The listing builds one solid part. Answer for the finished solid, in the listing's coordinates (mm). A direction names the side the tool comes from. Coordinates: 2 decimals unless noted, no trailing zeros. Order: outer loops, then holes, each group sorted by start corner. A loop starts at its lowest first (then second) coordinate and runs counter-clockwise, first axis right, second up. Notation, with made-up numbers: (61.5, 6) -> (81.5, 6) arc R14 ccw to (81.5, 19) -> close; hole circle Ø11 at (66, 7.25). An arc over 180 degrees is marked (long way). Put each result on its own line as item: value. Start each with the question number.
```python
from build123d import *

# Parameters (mm, degrees)
SKETCH_1_R              = 6.65
EXTRUDE_1_DEPTH         = 1.25
EXTRUDE_2_DEPTH         = 1.25
EXTRUDE_2_DEPTH_BACK    = 7
SKETCH_3_R              = 1.1
CUT_EXTRUDE_1_DEPTH     = 5
CHAMFER_1_SIZE          = 0.7
CUT_EXTRUDE1_DEPTH      = 10
CUT_EXTRUDE1_DEPTH_BACK = 10
SKETCH1_W               = 17.169793681
SKETCH1_H               = 8.928336681


with BuildPart() as part:
    # Эскиз1 → Бобышка-Вытянуть1 (new, symmetric)
    with BuildSketch(Plane(origin=(0, 0, 0), x_dir=(0, 0, -1), z_dir=(1, 0, 0))):
        with BuildLine():
            Line((-31.25, 0), (-10, 0))
            ThreePointArc((-10, 0), (-2.588190451, -9.659258263), (8.660254038, -5))
            Line((8.660254038, -5), (76.721847542, -5))
            ThreePointArc((76.721847542, -5), (75.425886146, -4.389181279), (74.09117429, -3.868451302))
            ThreePointArc((74.09117429, -3.868451302), (74.147561595, -2.912548148), (74.149130868, -1.954984622))
            ThreePointArc((74.149130868, -1.954984622), (75.638846987, -1.51744657), (77.087831178, -0.959648686))
            ThreePointArc((77.087831178, -0.959648686), (77.109856091, -0.006099484), (77.083941958, 0.947351948))
            ThreePointArc((77.083941958, 0.947351948), (75.643750299, 1.505844774), (74.166291118, 1.956600379))
            ThreePointArc((74.166291118, 1.956600379), (74.147505302, 2.913980899), (74.073940169, 3.8687157))
            ThreePointArc((74.073940169, 3.8687157), (75.433826566, 4.383081961), (76.750365892, 5))
            Line((76.750365892, 5), (8.660254038, 5))
            ThreePointArc((8.660254038, 5), (5, 8.660254038), (0, 10))
            Line((0, 10), (-34.75, 10))
            Line((-34.75, 10), (-34.75, 5))
            Line((-34.75, 5), (-35.25, 5))
            Line((-35.25, 5), (-35.25, 4))
            ThreePointArc((-35.25, 4), (-34.078427125, 1.171572875), (-31.25, 0))
        make_face()
        Circle(SKETCH_1_R, mode=Mode.SUBTRACT)
    extrude(amount=EXTRUDE_1_DEPTH, both=True)

    # Эскиз1<5> → Бобышка-Вытянуть2 (add, two sides: drawn at the far end of the back side and taken through both)
    with BuildSketch(Plane(origin=(0, 0, 0), x_dir=(0, 0, -1), z_dir=(1, 0, 0)).offset(-EXTRUDE_2_DEPTH_BACK)):
        with BuildLine():
            Line((73.559260736, 9.685830974), (74.227172899, 10))
            Line((74.227172899, 10), (80.32185029, 10))
            ThreePointArc((80.32185029, 10), (80.927765714, -1.515378033), (79.891173693, -13))
            Line((79.891173693, -13), (75.988629927, -13.007027449))
            ThreePointArc((75.988629927, -13.007027449), (76.159551637, -12.068663477), (76.283109214, -11.12289675))
            ThreePointArc((76.283109214, -11.12289675), (74.948016231, -10.345984286), (73.559260736, -9.669652694))
            ThreePointArc((73.559260736, -9.669652694), (73.690473514, -8.721120367), (73.767167518, -7.766631814))
            ThreePointArc((73.767167518, -7.766631814), (75.28662018, -7.447324325), (76.774901953, -7.004931935))
            ThreePointArc((76.774901953, -7.004931935), (76.871673579, -6.056050262), (76.920646267, -5.103504803))
            ThreePointArc((76.920646267, -5.103504803), (75.528713081, -4.433737489), (74.09117429, -3.868451302))
            ThreePointArc((74.09117429, -3.868451302), (74.147561595, -2.912548148), (74.149130868, -1.954984622))
            ThreePointArc((74.149130868, -1.954984622), (75.638846987, -1.51744657), (77.087831178, -0.959648686))
            ThreePointArc((77.087831178, -0.959648686), (77.109856091, -0.006099484), (77.083941958, 0.947351948))
            ThreePointArc((77.083941958, 0.947351948), (75.643750299, 1.505844774), (74.166291118, 1.956600379))
            ThreePointArc((74.166291118, 1.956600379), (74.147505302, 2.913980899), (74.073940169, 3.8687157))
            ThreePointArc((74.073940169, 3.8687157), (75.524735151, 4.421786748), (76.925488289, 5.091551117))
            ThreePointArc((76.925488289, 5.091551117), (76.872630699, 6.043888899), (76.771989513, 6.992367959))
            ThreePointArc((76.771989513, 6.992367959), (75.292418643, 7.436143003), (73.784148097, 7.769588967))
            ThreePointArc((73.784148097, 7.769588967), (73.691130431, 8.729989779), (73.559260736, 9.685830974))
        make_face()
    extrude(amount=EXTRUDE_2_DEPTH + EXTRUDE_2_DEPTH_BACK)

    # Эскиз3 → Вырез-Вытянуть1 (cut)
    with BuildSketch(Plane(origin=(0, 10, 0), x_dir=(1, 0, 0), z_dir=(0, 1, 0))):
        with Locations((0, -35)):
            Circle(SKETCH_3_R)
    extrude(amount=-CUT_EXTRUDE_1_DEPTH, mode=Mode.SUBTRACT)

    # Фаска1
    chamfer_1_edges = [part.edges().sort_by_distance(p)[0] for p in [
        (-1.25, 0, 6.65),
    ]]
    chamfer(chamfer_1_edges, length=CHAMFER_1_SIZE)

    # Sketch1 → Cut-Extrude1 (cut, two sides: drawn at the far end of the back side and taken through both)
    with BuildSketch(Plane(origin=(0, 0, 0), x_dir=(0, 0, -1), z_dir=(1, 0, 0)).offset(-CUT_EXTRUDE1_DEPTH_BACK)):
        with Locations((77.607372566, 9.464168341)):
            Rectangle(SKETCH1_W, SKETCH1_H)
    extrude(amount=CUT_EXTRUDE1_DEPTH + CUT_EXTRUDE1_DEPTH_BACK, mode=Mode.SUBTRACT)


solid = part.part
```
(1) A tool of negligible diameter and unlimited length cuts with its end or side. For faces 1 (the cylindrical face through (-2.93, -6.07, -76.87)), 2 (the cylindrical face through (-4.165, 4.375, -75.415)), 3 (the flat face through (0, 0, 21)), from which of +Z, -Z, +X, -X, +Y, -Y can it reach the whole face along a straight path? Write none if from no direction.
(2) The part is cut by section B-B on z = -66.5. Determine the outline of the cut face in (x, y), plus the area to 3 significant figures.
(3) Each of these flat-tipped pins is pushed along its axis until it touches: P1, Ø1.2, axis at x = 0.5, z = 21.5, coming from the -Y side; P2, Ø6, axis at y = -1, z = -24, coming from the -X side; P3, Ø1.2, axis at x = 0, z = -52, coming from the -Y side. Where does it stop, or does it pass through?
(4) The part is cut by section A-A on x = -5.5. Determine the outline of the cut face in (y, z).
(5) Find the intervals of material crossed by L1, parallel to X at y = 1.5, z = 25.5; L2, parallel to Y at x = 0.25, z = 13; L3, parallel to Z at x = -2.75, y = 0.25, in increasing order.
(6) For a pull along Y with two mould halves and no side action, classify faces 4 (the cylindrical face through (-2.93, -8.73, -73.69)), 5 (the flat face through (-1, 5, -47)), 6 (the cylindrical face through (0, 7.5, 33.9)) as released by +Y, released by -Y, zero draft, split by the parting line, or undercut.
Worked out:
1. face 1: +X, -X
1. face 2: +Z, -X, +Y
1. face 3: +Z, +X, -X, -Y
2. outline: (-1.25, -5) -> (1.25, -5) -> (1.25, 5) -> (-1.25, 5) -> close
2. area: 25.0 mm2
3. P1: y = 0
3. P2: x = -1.25
3. P3: y = -5
4. outline: (-13.01, -75.99) -> (-13, -79.89) arc R80.94 ccw to (5, -80.79) -> (5, -76.75) arc R18.99 cw to (3.87, -74.07) arc R16.72 cw to (1.96, -74.17) arc R20.93 cw to (0.95, -77.08) arc R18.98 cw to (-0.96, -77.09) arc R18.99 cw to (-1.95, -74.15) arc R16.72 cw to (-3.87, -74.09) arc R20.93 cw to (-5.1, -76.92) arc R18.98 cw to (-7, -76.77) arc R18.99 cw to (-7.77, -73.77) arc R16.72 cw to (-9.67, -73.56) arc R20.93 cw to (-11.12, -76.28) arc R18.98 cw to start
5. L1: -1.25 to 1.25
5. L2: 0 to 10
5. L3: -80.94 to -77.11
6. face 4: undercut
6. face 5: released by +Y
6. face 6: zero draft
